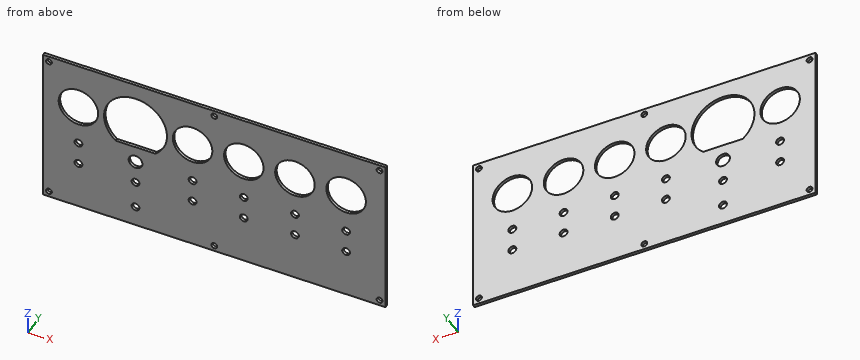
from build123d import *

# Parameters (mm, degrees)
F0_W     = 552.45
F0_H     = 260.35
F0_R     = 4.7625
F0_R_2   = 31.877
F1_DEPTH = 4.699
F2_R     = 6.35
F2_R_2   = 11.1125
F3_DEPTH = 25.4
F4_R     = 2.413
F5_DEPTH = 25.4


with BuildPart() as f1:
    # F0 (on Front) → F1 (new body)
    with BuildSketch(Plane.XZ):
        with Locations((15.887305, 34.925002)):
            Rectangle(F0_W, F0_H)
        with Locations((-250.812695, -85.724998)):
            Circle(F0_R, mode=Mode.SUBTRACT)
        with Locations((15.887305, -85.724998)):
            Circle(F0_R, mode=Mode.SUBTRACT)
        with Locations((282.587305, -85.724998)):
            Circle(F0_R, mode=Mode.SUBTRACT)
        with Locations((-203.187695, 88.900002)):
            Circle(F0_R_2, mode=Mode.SUBTRACT)
        with BuildLine():
            ThreePointArc((-143.233289, 49.543841), (-111.112695, 139.700002), (-78.9921, 49.543841))
            Line((-78.9921, 49.543841), (-143.233289, 49.543841))
        make_face(mode=Mode.SUBTRACT)
        with Locations((-19.037695, 88.900002)):
            Circle(F0_R_2, mode=Mode.SUBTRACT)
        with Locations((-250.812695, 155.575002)):
            Circle(F0_R, mode=Mode.SUBTRACT)
        with Locations((63.512305, 88.900002)):
            Circle(F0_R_2, mode=Mode.SUBTRACT)
        with Locations((146.062305, 88.900002)):
            Circle(F0_R_2, mode=Mode.SUBTRACT)
        with Locations((228.612305, 88.900002)):
            Circle(F0_R_2, mode=Mode.SUBTRACT)
        with Locations((15.887305, 155.575002)):
            Circle(F0_R, mode=Mode.SUBTRACT)
        with Locations((282.587305, 155.575002)):
            Circle(F0_R, mode=Mode.SUBTRACT)
    extrude(amount=-F1_DEPTH)

    # F2 (on face) → F3 (cut)
    with BuildSketch(Plane(origin=(0, 4.699, 0), x_dir=(-1, 0, 0), z_dir=(0, 1, 0))):
        with Locations((203.187695, 22.225002)):
            Circle(F2_R)
        with Locations((19.037695, 22.225002)):
            Circle(F2_R)
        with Locations((-63.512305, 22.225002)):
            Circle(F2_R)
        with Locations((-146.062305, 22.225002)):
            Circle(F2_R)
        with Locations((-228.612305, 22.225002)):
            Circle(F2_R)
        with Locations((203.187695, -15.874998)):
            Circle(F2_R)
        with Locations((19.037695, -15.874998)):
            Circle(F2_R)
        with Locations((-63.512305, -15.874998)):
            Circle(F2_R)
        with Locations((-146.062305, -15.874998)):
            Circle(F2_R)
        with Locations((-228.612305, -15.874998)):
            Circle(F2_R)
        with Locations((111.112695, -15.874998)):
            Circle(F2_R)
        with Locations((111.112695, 22.225002)):
            Circle(F2_R_2)
        with Locations((111.112695, -61.653677)):
            Circle(F2_R)
    extrude(amount=-F3_DEPTH, mode=Mode.SUBTRACT)

    # F4 (on face) → F5 (cut)
    with BuildSketch(Plane(origin=(0, 4.699, 0), x_dir=(-1, 0, 0), z_dir=(0, 1, 0))):
        with Locations((79.362695, 120.650002)):
            Circle(F4_R)
        with Locations((142.862695, 120.650002)):
            Circle(F4_R)
        with Locations((142.862695, 57.150002)):
            Circle(F4_R)
        with Locations((79.362695, 57.150002)):
            Circle(F4_R)
    extrude(amount=-F5_DEPTH, mode=Mode.SUBTRACT)


solid = f1.part
For this review, take the finished solid that the model builds, in its own axes (mm). Round coordinates to 2 decimals unless told otherwise and drop trailing zeros. Loops run counter-clockwise (first coordinate to the right, second up) from the corner with the lowest first, then second, coordinate; pieces in that order, holes last. Notation, with made-up numbers: (81, 63.25) - (100, 63.25) arc R16 cw to (100, 81.25) - close; hole circle Ø10 at (-13, 33.25). An arc over 180 degrees is marked (long way). Put each result on its own line as item: value. Start each with the question number.
1. Consider section C-C on z = 134. State the section outline as (x, y) points.
2. For probe 1 along Z at (x, y) = (-23.5, 4.2); probe 2 along Z at (x, y) = (53, 3.75); probe 3 along Z at (x, y) = (-42, 0.85), list the stretches that pass through material, from the lowest coordinate up. Write a range as [from, to].
3. Insertion check: P1, Ø10, axis at x = -19.04, z = 22.23, coming from the -Y side; P2, Ø16.5, axis at x = -19.04, z = -15.87, coming from the +Y side. Each pin has a flat end and moves straight along its axis. Give the tip position at first contact, or say it passes through.
4. Consider section B-B on x = -93. State the section outline as (y, z) points.
5. Consider section A-A on z = 75.5. State the section outline as (x, y) points.
6. Consider section D-D on y = 1.95. State how many separate pieces and enclosed holes the cut face has, plus the area to 3 significant figures.
Result sheet:
1. outline: (-260.34, 0) - (-134.49, 0) - (-134.49, 4.7) - (-260.34, 4.7) - close; (-87.73, 0) - (292.11, 0) - (292.11, 4.7) - (-87.73, 4.7) - close
2. probe 1: [-95.25, -20.39], [-11.36, 17.71], [26.74, 57.34], [120.46, 165.1]
2. probe 2: [-95.25, 58.81], [118.99, 165.1]
2. probe 3: [-95.25, 66.79], [111.01, 165.1]
3. P1: through
3. P2: y = 4.7
4. outline: (0, -95.25) - (4.7, -95.25) - (4.7, 49.54) - (0, 49.54) - close; (0, 136.36) - (4.7, 136.36) - (4.7, 165.1) - (0, 165.1) - close
5. outline: (-260.34, 0) - (-232.11, 0) - (-232.11, 4.7) - (-260.34, 4.7) - close; (-174.26, 0) - (-160.11, 0) - (-160.11, 4.7) - (-174.26, 4.7) - close; (-62.11, 0) - (-47.96, 0) - (-47.96, 4.7) - (-62.11, 4.7) - close; (9.89, 0) - (34.59, 0) - (34.59, 4.7) - (9.89, 4.7) - close; (92.44, 0) - (117.14, 0) - (117.14, 4.7) - (92.44, 4.7) - close; (174.99, 0) - (199.69, 0) - (199.69, 4.7) - (174.99, 4.7) - close; (257.54, 0) - (292.11, 0) - (292.11, 4.7) - (257.54, 4.7) - close
6. separate pieces: 1
6. enclosed holes: 25
6. area: 118,000 mm^2
